```python
from build123d import *

# Parameters (mm, degrees)
BOSS_EXTRUDE1_DEPTH = 16
SKETCH2_R           = 1.25
CUT_EXTRUDE1_DEPTH  = 10
CUT_EXTRUDE2_REACH  = 24.5
SKETCH4_R           = 1.25
FILLET1_R           = 1.5
SKETCH8_W           = 29
SKETCH8_H           = 3
CUT_EXTRUDE3_DEPTH  = 10


with BuildPart() as part:
    # Sketch1 → Boss-Extrude1 (new body)
    with BuildSketch(Plane.XY):
        Polygon((-32.25, 0), (-32.25, -3.15), (-25, -3.15), (-25, -10.5), (25, -10.5), (25, -3.15), (32.25, -3.15), (32.25, 0), (25, 0), (25, 3), (35.25, 3), (35.25, -6.15), (28, -6.15), (28, -13.5), (21.5, -13.5), (21.5, -19.5), (14.5, -19.5), (14.5, -13.5), (-14.5, -13.5), (-14.5, -19.5), (-21.5, -19.5), (-21.5, -13.5), (-28, -13.5), (-28, -6.15), (-35.25, -6.15), (-35.25, 3), (-25, 3), (-25, 0), align=None)
    extrude(amount=BOSS_EXTRUDE1_DEPTH)

    # Sketch2 → Cut-Extrude1 (cut, through all)
    with BuildSketch(Plane(origin=(0, -10.5, 0), x_dir=(1, 0, 0), z_dir=(0, 1, 0))):
        with Locations((-18, -3.5)):
            Circle(SKETCH2_R)
        with Locations((18, -3.5)):
            Circle(SKETCH2_R)
    extrude(amount=-CUT_EXTRUDE1_DEPTH, mode=Mode.SUBTRACT)

    # Sketch4 → Cut-Extrude2 (cut, up to next)
    with BuildSketch(Plane(origin=(0, 3, 0), x_dir=(1, 0, 0), z_dir=(0, 1, 0)), mode=Mode.PRIVATE) as cut_extrude2_sk1:
        with Locations((-28.625, -8)):
            Circle(SKETCH4_R)
    cut_extrude2_tool1 = extrude(cut_extrude2_sk1.sketch, amount=-CUT_EXTRUDE2_REACH, mode=Mode.PRIVATE) & part.part
    add(cut_extrude2_tool1.solids().sort_by_distance((-28.625, 3, 8))[0], mode=Mode.SUBTRACT)
    # Sketch4 → Cut-Extrude2 (cut, up to next)
    with BuildSketch(Plane(origin=(0, 3, 0), x_dir=(1, 0, 0), z_dir=(0, 1, 0)), mode=Mode.PRIVATE) as cut_extrude2_sk2:
        with Locations((28.625, -8)):
            Circle(SKETCH4_R)
    cut_extrude2_tool2 = extrude(cut_extrude2_sk2.sketch, amount=-CUT_EXTRUDE2_REACH, mode=Mode.PRIVATE) & part.part
    add(cut_extrude2_tool2.solids().sort_by_distance((28.625, 3, 8))[0], mode=Mode.SUBTRACT)

    # Fillet1
    fillet1_edges = [part.edges().sort_by_distance(p)[0] for p in [
        (-25, -10.5, 8),
        (25, -10.5, 8),
        (25, 3, 8),
        (35.25, 3, 8),
        (35.25, -6.15, 8),
        (28, -6.15, 8),
        (28, -13.5, 8),
        (21.5, -13.5, 8),
        (21.5, -19.5, 8),
        (14.5, -19.5, 8),
        (-14.5, -19.5, 8),
        (-21.5, -19.5, 8),
        (-21.5, -13.5, 8),
        (-28, -13.5, 8),
        (-28, -6.15, 8),
        (-35.25, -6.15, 8),
        (-35.25, 3, 8),
        (-25, 3, 8),
    ]]
    fillet(fillet1_edges, radius=FILLET1_R)

    # Sketch8 → Cut-Extrude3 (cut, through all)
    with BuildSketch(Plane(origin=(0, -10.5, 0), x_dir=(1, 0, 0), z_dir=(0, 1, 0))):
        with Locations((0, -14.5)):
            Rectangle(SKETCH8_W, SKETCH8_H)
    extrude(amount=-CUT_EXTRUDE3_DEPTH, mode=Mode.SUBTRACT)


solid = part.part
```
Check sheet for the modelled part. Datum: model origin and axes. Units: mm. A direction names the side the tool comes from. Round coordinates to 2 decimals unless told otherwise and drop trailing zeros. Loops run counter-clockwise (first coordinate to the right, second up) from the corner with the lowest first, then second, coordinate; pieces in that order, holes last. Notation, with made-up numbers: (68.25, 27) -> (79.25, 27) arc R24 cw to (79.25, 44) -> close; hole circle Ø4 at (79.5, 29.25). An arc over 180 degrees is marked (long way). Write item = value, one per line. Start each with the question number.
1) Thickness scan on probe 1 along X at (y, z) = (-16.25, 3.5); probe 2 along X at (y, z) = (1.2, 8) (3 decimals); probe 3 along X at (y, z) = (-11.25, 14). Record the ranges inside material, lowest first.
2) Set-up check for faces 4 (the cylindrical face through (24.55, -10.07, 8.11)), 5 (the cylindrical face through (14.95, -19.07, 8.11)), 6 (the flat face through (32.25, -2, 8)), 7 (the flat face through (-32, -6.15, 8)), 8 (the flat face through (28, -10, 8)): record each of +Z, -Z, +X, -X, +Y, -Y from which the full face is reachable in a straight line by a thin tool's end or side.
3) Sectioned sample at C-C, the plane x = -10.5. Record the cut outline in (y, z), plus the area to 3 significant figures.
4) Gauge pin test, flat ends, axial feed: pin 1 Ø2 at (y, z) = (-15.5, 14) entering from -X; pin 2 Ø4 at (x, z) = (-24.5, 12) entering from -Y; pin 3 Ø1 at (x, z) = (0, 2) entering from -Y. Record the tip position at first contact, or that the pin passes through.
5) Sectioned sample at B-B, the plane z = 3.5. State how many separate pieces and enclosed holes the cut face has, plus the area to 3 significant figures.
6) Sectioned sample at A-A, the plane x = 18. Record the cut outline in (y, z).
7) Sectioned sample at D-D, the plane x = -18.5. Record the cut outline in (y, z), plus the area to 3 significant figures.
8) Release check for a two-part mould opening along X. For faces 1 (the cylindrical face through (34.82, -5.7, 8.11)), 2 (the flat face through (-25, 1, 8)), 3 (the flat face through (-28, -10, 8)) record: released by +X, released by -X, zero draft, split by the parting line, or undercut.
Results are:
q1.probe_1 = -21.5 to -19.25, -16.75 to -14.5, 14.5 to 16.75, 19.25 to 21.5
q1.probe_2 = -35.25 to -29.875, -27.375 to -25, 25 to 27.375, 29.875 to 35.25
q1.probe_3 = -28 to -14.5, 14.5 to 28
q2.face_4 = +Z, -Z, +Y
q2.face_5 = +Z, -Z, -Y
q2.face_6 = +Z, -Z
q2.face_7 = +Z, -Z, -X, -Y
q2.face_8 = +Z, -Z, +X, -Y
q3.outline = (-13.5, 0) -> (-10.5, 0) -> (-10.5, 13) -> (-13.5, 13) -> close
q3.area = 39.0 mm^2
q4.pin_1 = -21.59
q4.pin_2 = -13.59
q4.pin_3 = -13.5
q5.separate_pieces = 3
q5.enclosed_holes = 0
q5.area = 372 mm^2
q6.outline = (-19.5, 0) -> (-10.5, 0) -> (-10.5, 2.25) -> (-19.5, 2.25) -> close; (-19.5, 4.75) -> (-10.5, 4.75) -> (-10.5, 16) -> (-19.5, 16) -> close
q7.outline = (-19.5, 0) -> (-10.5, 0) -> (-10.5, 2.35) -> (-19.5, 2.35) -> close; (-19.5, 4.65) -> (-10.5, 4.65) -> (-10.5, 16) -> (-19.5, 16) -> close
q7.area = 123 mm^2
q8.face_1 = released by +X
q8.face_2 = undercut
q8.face_3 = released by -X
